from build123d import *

# Parameters (mm, degrees)
F0_R      = 16
F1_DEPTH  = 2
F2_SIZE   = 1
F4_R      = 15
F5_DEPTH  = 13
F6_R      = 16
F7_DEPTH  = 1
F8_SIZE   = 0.99999
F9_DEPTH  = 1
F10_R     = 1.25
F11_DEPTH = 2.5
F12_D     = 2.5


# Not quite as in the source:
# - a fillet or chamfer is up to 0.001 mm smaller than in the source, because OpenCascade refuses the exact size


with BuildPart() as f1:
    # F0 (on Top) → F1 (new body)
    with BuildSketch(Plane.XY):
        Circle(F0_R)
    extrude(amount=F1_DEPTH)

    # F2
    f2_edges = [f1.edges().sort_by_distance(p)[0] for p in [
        (-16, 0, 2),
    ]]
    chamfer(f2_edges, length=F2_SIZE)

    # F4 (on face) → F5 (join)
    with BuildSketch(Plane.XY.offset(2)):
        Circle(F4_R)
    extrude(amount=F5_DEPTH)

    # F6 (on face) → F7 (join)
    with BuildSketch(Plane.XY.offset(15)):
        Circle(F6_R)
    extrude(amount=F7_DEPTH)

    # F8 (size 1 in the source; OpenCascade refuses exactly that, so slightly less here)
    f8_edges = [f1.edges().sort_by_distance(p)[0] for p in [
        (-16, 0, 15),
    ]]
    chamfer(f8_edges, length=F8_SIZE)

    # F9 (add): a face of the model
    f9_faces = [f1.faces().sort_by_distance(p)[0] for p in [
        (0, 0, 16),
    ]]
    extrude(f9_faces, amount=F9_DEPTH)

    # F10 (on face) → F11 (cut)
    with BuildSketch(Plane.XY):
        Circle(F10_R)
    extrude(amount=-F11_DEPTH, mode=Mode.SUBTRACT)

    # F12 (through all)
    with Locations(Plane(origin=(0, 0, 0), x_dir=(1, 0, 0), z_dir=(0, 0, -1))):
        with Locations((0, 0)):
            Hole(F12_D / 2)


solid = f1.part
The model under review builds one solid part; all positions refer to its coordinate system, in mm. A direction names the side the tool comes from. Give positions to 0.01 mm unless a question says otherwise; leave off trailing zeros. Order: outer loops, then holes, each group sorted by start corner. A loop starts at its lowest first (then second) coordinate and runs counter-clockwise, first axis right, second up. Notation, with made-up numbers: (5, -6) -> (35, -6) arc R17 cw to (35, 27) -> close; hole circle Ø2 at (-2.75, 46.25). An arc over 180 degrees is marked (long way). Write item = value, one per line. Start each with the question number.
(1) Take a section at C-C (z = 9.25). Write out the cut boundary in (x, y), plus the area to 3 significant figures.
(2) For pin 1 Ø10 at (x, z) = (-10, 11.5) entering from +Y; pin 2 Ø8 at (x, y) = (-1, -0.5) entering from -Z; pin 3 Ø5 at (y, z) = (-5, 3) entering from +X; pin 4 Ø6 at (y, z) = (12, 11.5) entering from -X, all flat-tipped, find the tip position at first contact; note any pin that passes through.
(3) For L1, parallel to Y at x = 0, z = 6.5; L2, parallel to X at y = -1, z = 2.75; L3, parallel to X at y = 0.5, z = 10.25, list the stretches that pass through material, from the lowest coordinate up. Write a range as from..to.
(4) Draft analysis for pull direction Y (two halves, no side actions). For faces 1 (the cylindrical face through (0.27, 1.22, 8.62)), 2 (the flat face through (3, 0, 0)), 3 (the cylindrical face through (-3.47, -15.62, 16.49)), state which applies: +Y half, -Y half, draft (parallel to the pull), parting line (faces both ways), or undercut.
(5) Tool access review of faces 4 (the cylindrical face through (-3.47, -15.62, 0.49)), 5 (the cylindrical face through (-14.985, 0.66, 8.409)): name each direction out of +Z, -Z, +X, -X, +Y, -Y from which nothing blocks a thin tool from reaching the whole face with its end or side.
Returned:
q1.outline = circle Ø30 at (0, 0); hole circle Ø2.5 at (0, 0)
q1.area = 702 mm²
q2.pin_1 = 14.14
q2.pin_2 = 0
q2.pin_3 = 15.61
q2.pin_4 = -12
q3.L1 = -15..-1.25, 1.25..15
q3.L2 = -14.97..-0.75, 0.75..14.97
q3.L3 = -14.99..-1.15, 1.15..14.99
q4.face_1 = undercut
q4.face_2 = draft
q4.face_3 = parting line
q5.face_4 = +Z, -Z
q5.face_5 = none
